Could you check a few things on this model? Use its own coordinates, in mm. Face numbers are marked on the shaded views. A direction names the side the tool comes from. Round coordinates to 2 decimals unless told otherwise and drop trailing zeros. Loops run counter-clockwise (first coordinate to the right, second up) from the corner with the lowest first, then second, coordinate; pieces in that order, holes last. Notation, with made-up numbers: (79, 58) -> (86, 58) arc R24 cw to (86, 75) -> close; hole circle Ø5 at (62, 20). An arc over 180 degrees is marked (long way). One line per item, written item: value.
Autodesk Fusion 360 part; units mm, degrees
sketch "Sketch1" plane through (0, 0, 0) normal (0, 0, 1) x (1, 0, 0)
  circle A0 centre (0, 0) radius 6
  dimension "d1" = 12
extrude "Extrude1" add sketch "Sketch1" along normal blind 3
sketch "Sketch2" plane through (0, 0, 3) normal (0, 0, 1) x (-1, 0, 0)
  circle A0 centre (0, 0) radius 6
  circle A1 centre (0, 0) radius 3.5
  dimension "d4" = 7
extrude "Extrude2" add sketch "Sketch2" along normal blind 8 contours A1
sketch "Sketch3" plane through (0, 0, 11) normal (0, 0, 1) x (-1, 0, 0)
  circle A0 centre (0, 0) radius 3.5
  circle A1 centre (0, 0) radius 2.4
  dimension "d7" = 4.8
extrude "Extrude3" add sketch "Sketch3" along normal blind 5.2 contours A1
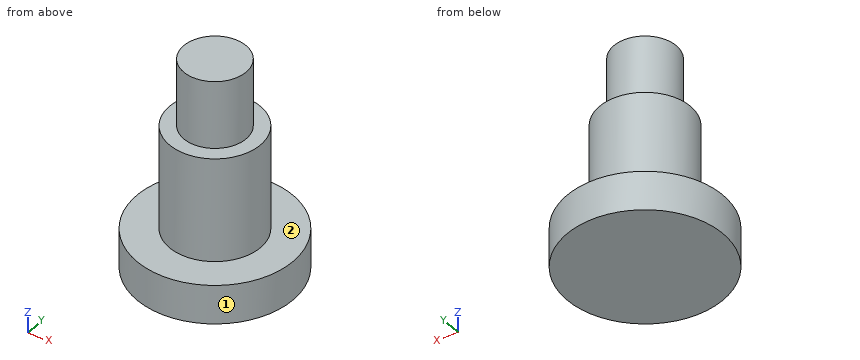
(1) If I drill on L1, parallel to Z at x = -4, y = -1.5; L2, parallel to Y at x = 0, z = 10.5; L3, parallel to Z at x = 2.5, y = -0.5, over which ranges is the centre line in solid material (lowest first)?
Recorded:
L1: 0 to 3
L2: -3.5 to 3.5
L3: 0 to 11
(2) I'm going to push flat-ended pins straight in: pin 1 Ø2 at (y, z) = (-4.5, 3.5) entering from -X; pin 2 Ø1 at (x, z) = (2, 9) entering from +Y; pin 3 Ø5 at (x, z) = (-1, 6) entering from -Y. Where does each tip first touch, or does it pass through?
Recorded:
pin 1: x = -4.77
pin 2: y = 3.16
pin 3: y = -3.5
(3) If we section it at A-A, the plane x = 0: Please give me the cut outline in (y, z), then the cut area to 3 significant figures.
Recorded:
outline: (-6, 0) -> (6, 0) -> (6, 3) -> (3.5, 3) -> (3.5, 11) -> (2.4, 11) -> (2.4, 16.2) -> (-2.4, 16.2) -> (-2.4, 11) -> (-3.5, 11) -> (-3.5, 3) -> (-6, 3) -> close
area: 117 mm²
(4) If we section it at C-C, the plane z = 11.25: Please give me the cut outline in (x, y).
Recorded:
outline: circle Ø4.8 at (0, 0)
(5) If we section it at D-D, the plane x = -3: Please give me the cut outline in (y, z).
Recorded:
outline: (-5.2, 0) -> (5.2, 0) -> (5.2, 3) -> (1.8, 3) -> (1.8, 11) -> (-1.8, 11) -> (-1.8, 3) -> (-5.2, 3) -> close
(6) For the marked faces 1 and 2, which set-ups out of +Z, -Z, +X, -X, +Y, -Y let a thin tool reach every point of the face, with its end or its side?
Recorded:
face 1: +Z, -Z
face 2: +Z
